Geometry check sheet. Reference: drawing and pictorial views, mm from the part's lowest x, y, z. Coordinates: 2 decimals unless noted, no trailing zeros. Write each loop counter-clockwise with the first axis right and the second up, starting at its lowest first coordinate (ties: lowest second). Pieces come first, ordered by that corner, then holes. Notation, with made-up numbers: (12, 28.25) - (28, 28.25) arc R6 cw to (28, 35.25) - close; hole circle Ø7 at (79, 18). An arc over 180 degrees is marked (long way). Use one line per item in the form item = value. Start each with the question number.
(1) Gauge pin test, flat ends, axial feed: pin 1 Ø4 at (x, z) = (6, 94.5) entering from -Y; pin 2 Ø2 at (x, y) = (11, 10.5) entering from +Z. Record the tip position at first contact, or that the pin passes through.
(2) Material ranges on line 1 (Z direction, x = 4.75, y = 11); line 2 (Z direction, x = 1.75, y = 12.25), recorded low to high. Write a range as [from, to].
(3) Sectioned sample at A-A (x = 1.75). Record the cut outline in (y, z), and give its area (3 significant figures).
(4) Sectioned sample at B-B (y = 11.75). Record the cut outline in (x, z).
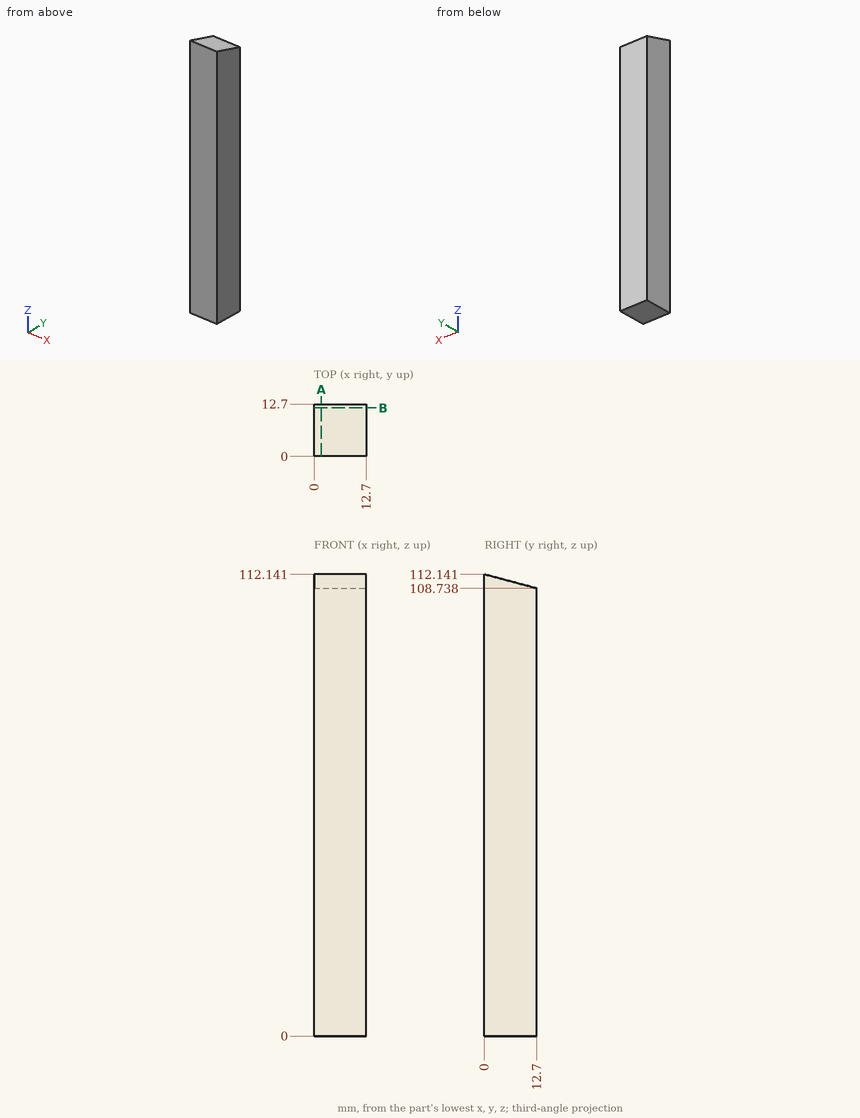
Answers below:
q1.pin_1 = 0
q1.pin_2 = 109.6
q2.line_1 = [0, 109.19]
q2.line_2 = [0, 108.86]
q3.outline = (0, 0) - (12.7, 0) - (12.7, 108.74) - (0, 112.14) - close
q3.area = 1,400 mm2
q4.outline = (0, 0) - (12.7, 0) - (12.7, 108.99) - (0, 108.99) - close
